For this review, take the finished solid that the model builds, in its own axes (mm). Face numbers are marked on the shaded views. Coordinates: 2 decimals unless noted, no trailing zeros. Loops run counter-clockwise (first coordinate to the right, second up) from the corner with the lowest first, then second, coordinate; pieces in that order, holes last. Notation, with made-up numbers: (12, -36) -> (71, -36) arc R8 ccw to (71, -32) -> close; hole circle Ø7 at (-22.75, 20). An arc over 180 degrees is marked (long way). Use a Markdown table: item, result.
from build123d import *
from build123d.topology import SkipClean

# Parameters (mm, degrees)
SKETCH_2_R               = 3
CUT_EXTRUDE_1_DEPTH      = 6
CUT_EXTRUDE_2_DEPTH      = 20.756862782
CUT_EXTRUDE_2_DEPTH_BACK = 20.756862782


with BuildPart() as part:
    # Эскиз1 → Повернуть1 (revolve)
    with BuildSketch(Plane.XY):
        Polygon((-9.432089165, 2.077253219), (-9.432089165, 9.077253219), (-8.432089165, 9.077253219), (-8.432089165, 6.077253219), (-7.432089165, 6.077253219), (-7.432089165, 9.077253219), (-6.432089165, 9.077253219), (-6.432089165, 8.562024792), (-5.432089165, 9.577253219), (1.567910835, 9.577253219), (3.567910835, 7.607253219), (15.567910835, 7.607253219), (15.567910835, 2.077253219), align=None)
    revolve(axis=Axis((15.567910835, 2.077253219, 0), (-1, 0, 0)))

    # Эскиз2 → Вырез-Вытянуть1 (cut)
    with BuildSketch(Plane.ZY.offset(9.432089165)):
        with Locations(Location((0, 2.077253219, 0), (0, 0, 270))):
            Circle(SKETCH_2_R)
    extrude(amount=-CUT_EXTRUDE_1_DEPTH, mode=Mode.SUBTRACT)

    # Эскиз3 → Вырез-Вытянуть2 (cut, two sides: drawn at the far end of the back side and taken through both)
    with SkipClean():  # the faces are left unmerged after this step: merging them gives an invalid solid
        with BuildSketch(Plane(origin=(0, 0, 0), x_dir=(1, 0, 0), z_dir=(0, 1, 0)).offset(-CUT_EXTRUDE_2_DEPTH_BACK)):
            Polygon((3.567910835, -5.53), (14.748858559, 5.650947724), (16.371941026, 5.650947724), (16.371941026, -6.819604623), (3.567910835, -5.789196512), align=None)
        extrude(amount=CUT_EXTRUDE_2_DEPTH + CUT_EXTRUDE_2_DEPTH_BACK, mode=Mode.SUBTRACT)


solid = part.part
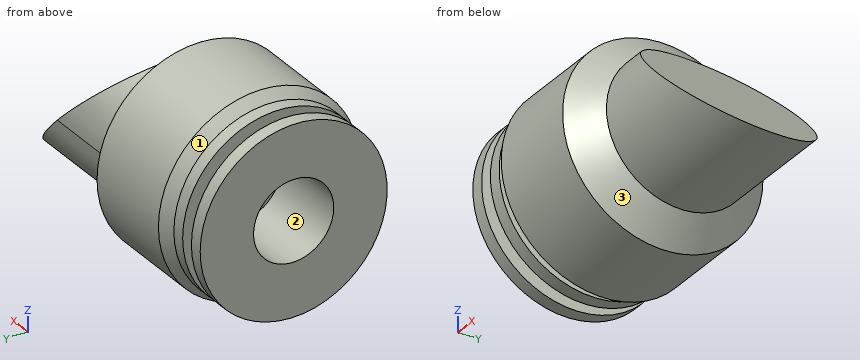
(1) Mouldability with a two-part tool opening along X and no side actions: class the marked faces 1, 2 and 3 as pulls with the +X half, pulls with the -X half, needs draft (parallel to the pull), parting line crosses it, or undercut.
Found:
| item | result |
|---|---|
| face 1 | undercut |
| face 2 | needs draft |
| face 3 | pulls with the +X half |
(2) Take a section at B-B on x = -3. Write out the cut boundary in (y, z).
Found:
| item | result |
|---|---|
| outline | circle Ø15 at (2.08, 0) |
(3) For line 1 along X through (y, z) = (0.5, -6.5); line 2 along X through (y, z) = (1, 6.75); line 3 along X through (y, z) = (-4, 2), list the stretches that pass through material, from the lowest coordinate up.
Found:
| item | result |
|---|---|
| line 1 | x = -9.43 to -8.43, -7.43 to -6.43, -6.23 to 2.39 |
| line 2 | x = -9.43 to -8.43, -7.43 to -6.43, -6.09 to 2.24 |
| line 3 | x = -9.43 to -8.43, -7.43 to 2.69 |
(4) Take a section at A-A on x = -7. Write out the cut boundary in (y, z), plus the area to 3 significant figures.
Found:
| item | result |
|---|---|
| outline | circle Ø14 at (2.08, 0); hole circle Ø6 at (2.08, 0) |
| area | 126 mm^2 |
(5) For pin 1 Ø6 at (x, y) = (9, 4) entering from -Z; pin 2 Ø8 at (x, y) = (10, 1.5) entering from +Z; pin 3 Ø3 at (x, y) = (10, -3.5) entering from +Z; pin 4 Ø6.5 at (y, z) = (1, 0.5) entering from -X, all flat-tipped, find the tip position at first contact; note any pin that passes through.
Found:
| item | result |
|---|---|
| pin 1 | stops at z = -5.53 |
| pin 2 | stops at z = 3.1 |
| pin 3 | stops at z = 0.6 |
| pin 4 | stops at x = -9.43 |
